Could you check a few things on this drawing? It's one solid part, dimensions in mm from its lowest x, y, z. A direction names the side the tool comes from. Give positions to 0.01 mm unless a question says otherwise; leave off trailing zeros. Loops run counter-clockwise (first coordinate to the right, second up) from the corner with the lowest first, then second, coordinate; pieces in that order, holes last. Notation, with made-up numbers: (78.5, 54.5) - (120.5, 54.5) arc R21 cw to (120.5, 67.5) - close; hole circle Ø6 at (3.5, 78.25). An arc over 180 degrees is marked (long way). Write item = value, one per line.
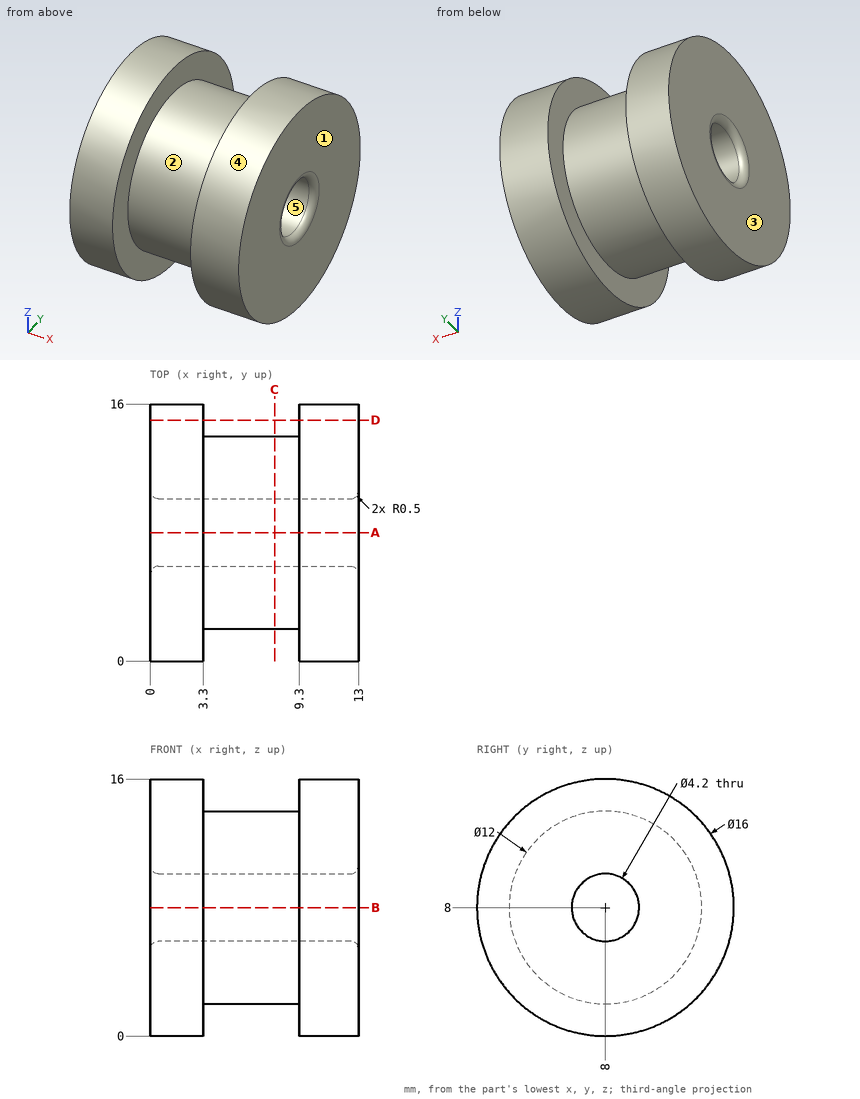
Q1. Which directions (+Z, -Z, +X, -X, +Y, -Y) give clear straight access to the entire face, cutting with the end or side of a thin tool? Please do the marked faces 1 and 2.
Output:
face_1 = +Z, -Z, +X, +Y, -Y
face_2 = none
Q2. We'd pull the mould along Z, two halves only. Please class the marked faces 3, 4 and 5: released by +Z, released by -Z, zero draft, split by the parting line, or undercut.
Output:
face_3 = zero draft
face_4 = split by the parting line
face_5 = undercut
Q3. Imagine slicing it at D-D, the plane y = 15. Write out the boundary of the cut face in (x, z).
Output:
outline = (0, 4.13) - (3.3, 4.13) - (3.3, 11.87) - (0, 11.87) - close; (9.3, 4.13) - (13, 4.13) - (13, 11.87) - (9.3, 11.87) - close
Q4. For pin 1 (5 mm diameter, centred on x = 6.5, y = 3, fed in from +Z); pin 2 (4 mm diameter, centred on x = 6.5, z = 6.5, fed in from +Y); pin 3 (1.5 mm diameter, centred on x = 7, z = 7, fed in from -Y), each with a flat end and sliding along its axis, tell me the tip position at first contact or that it passes through.
Output:
pin_1 = 13.45
pin_2 = 14
pin_3 = 2.01
Q5. Imagine slicing it at A-A, the plane y = 8. Write out the boundary of the cut face in (x, z).
Output:
outline = (0, 0) - (3.3, 0) - (3.3, 2) - (9.3, 2) - (9.3, 0) - (13, 0) - (13, 5.4) arc R0.5 ccw to (12.5, 5.9) - (0.5, 5.9) arc R0.5 ccw to (0, 5.4) - close; (0, 10.6) arc R0.5 ccw to (0.5, 10.1) - (12.5, 10.1) arc R0.5 ccw to (13, 10.6) - (13, 16) - (9.3, 16) - (9.3, 14) - (3.3, 14) - (3.3, 16) - (0, 16) - close
Q6. Imagine slicing it at C-C, the plane x = 7.75. Write out the boundary of the cut face in (y, z), then the cut area to 3 significant figures.
Output:
outline = circle Ø12 at (8, 8); hole circle Ø4.2 at (8, 8)
area = 99.2 mm2
Q7. I need wall thicknesses on L1, parallel to X at y = 5.5, z = 14.25; L2, parallel to Y at x = 4.5, z = 8; L3, parallel to Y at x = 3, z = 8. Which ranges of each line are inside material? Lowest first, please.
Output:
L1 = 0 to 3.3, 9.3 to 13
L2 = 2 to 5.9, 10.1 to 14
L3 = 0 to 5.9, 10.1 to 16
